The listing builds one solid part. Answer for the finished solid, in the listing's coordinates (mm). Face numbers are marked on the shaded views. A direction names the side the tool comes from. Coordinates: 2 decimals unless noted, no trailing zeros. Order: outer loops, then holes, each group sorted by start corner. A loop starts at its lowest first (then second) coordinate and runs counter-clockwise, first axis right, second up. Notation, with made-up numbers: (1, 59.25) -> (15, 59.25) arc R22 ccw to (15, 96.25) -> close; hole circle Ø9 at (21, 6.25). An arc over 180 degrees is marked (long way). Answer in a Markdown table with one row per item. Add a question column.
```python
from build123d import *

# Parameters (mm, degrees)
RESSALTO_EXTRUS_O1_DEPTH = 10
ESBO_O3_R                = 1.5
CORTE_EXTRUS_O1_DEPTH    = 10


with BuildPart() as part:
    # Esboço2 → Ressalto-extrusão1 (new body)
    with BuildSketch(Plane.XY):
        with BuildLine():
            Line((-2.16273614, 4.130820826), (4.83726386, 4.130820826))
            ThreePointArc((4.83726386, 4.130820826), (6.687556539, 1.360164653), (7.33726386, -1.907556116))
            Line((7.33726386, -1.907556116), (7.33726386, -5.469179174))
            Line((7.33726386, -5.469179174), (14.33726386, -5.469179174))
            Line((14.33726386, -5.469179174), (14.33726386, -3.493237638))
            Line((14.33726386, -3.493237638), (9.33726386, -3.493237638))
            Line((9.33726386, -3.493237638), (9.33726386, -0.739966657))
            ThreePointArc((9.33726386, -0.739966657), (8.579234613, 2.826995847), (6.436166726, 5.777434776))
            Line((6.436166726, 5.777434776), (-3.761639005, 5.777434776))
            ThreePointArc((-3.761639005, 5.777434776), (-5.904706893, 2.826995847), (-6.66273614, -0.739966657))
            Line((-6.66273614, -0.739966657), (-6.66273614, -3.493237638))
            Line((-6.66273614, -3.493237638), (-11.66273614, -3.493237638))
            Line((-11.66273614, -3.493237638), (-11.66273614, -5.469179174))
            Line((-11.66273614, -5.469179174), (-4.66273614, -5.469179174))
            Line((-4.66273614, -5.469179174), (-4.66273614, -1.907556116))
            ThreePointArc((-4.66273614, -1.907556116), (-4.013028819, 1.360164653), (-2.16273614, 4.130820826))
        make_face()
    extrude(amount=RESSALTO_EXTRUS_O1_DEPTH)

    # Esboço3 → Corte-extrusão1 (cut)
    with BuildSketch(Plane(origin=(0, -3.493237638, 0), x_dir=(1, 0, 0), z_dir=(0, 1, 0))):
        with Locations(Location((-9.16273614, -5, 0), (0, 0, 270))):
            Circle(ESBO_O3_R)
        with Locations(Location((11.83726386, -5, 0), (0, 0, 180))):
            Circle(ESBO_O3_R)
    extrude(amount=-CORTE_EXTRUS_O1_DEPTH, mode=Mode.SUBTRACT)


solid = part.part
```
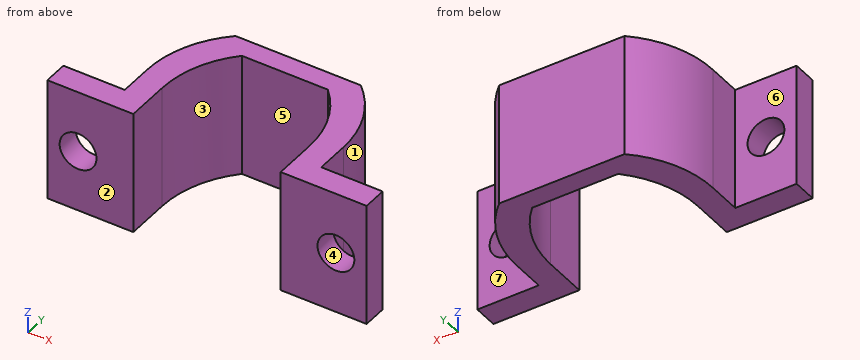
Q1. For the marked faces 4, 5, 6 and 7, determine the directions among +Z, -Z, +X, -X, +Y, -Y from which every point of the face is accessible in a straight line to the end or side of a thin tool.
Q2. A cutting plane is placed at C-C (z = 9.25). Determine the outline of the cut face in (x, y), then the cut area to 3 significant figures.
Q3. Straight lines are drawn through the part: line 1 (X direction, y = -3.25, z = 9.75); line 2 (X direction, y = -4.5, z = 8.5); line 3 (X direction, y = -4, z = 6.25). For each, find the intervals that lie inside material, in ascending order.
Q4. A cutting plane is placed at B-B (y = -3.25). Determine the outline of the cut face in (x, z).
Q5. Given pin 1 (2 mm diameter, centred on y = -1.5, z = 4, fed in from -X); pin 2 (6 mm diameter, centred on x = -1.5, y = -2.5, fed in from -Z); pin 3 (2 mm diameter, centred on y = -2, z = 6.5, fed in from +X); pin 4 (5.5 mm diameter, centred on x = -8, z = 7.5, fed in from +Y), each flat-ended and moving along its own axis, determine where each tip first touches the part or whether it passes through.
Q6. A cutting plane is placed at A-A (z = 5). Determine the outline of the cut face in (x, y), then the cut area to 3 significant figures.
Q7. A cutting plane is placed at D-D (x = -0.75). Determine the outline of the cut face in (y, z), then the cut area to 3 significant figures.
Q8. Determine the mould class of the marked faces 1, 2 and 3 for opening direction X: +X half, -X half, draft (parallel to the pull), parting line (faces both ways), or undercut.
Returned:
| question | item | result |
|---|---|---|
| 1 | face 4 | +Y, -Y |
| 1 | face 5 | +Z, -Z, -Y |
| 1 | face 6 | +Z, -Z, -X, +Y |
| 1 | face 7 | +Z, -Z, +X, +Y |
| 2 | outline | (-11.66, -5.47) -> (-4.66, -5.47) -> (-4.66, -1.91) arc R8.54 cw to (-2.16, 4.13) -> (4.84, 4.13) arc R8.54 cw to (7.34, -1.91) -> (7.34, -5.47) -> (14.34, -5.47) -> (14.34, -3.49) -> (9.34, -3.49) -> (9.34, -0.74) arc R8.77 ccw to (6.44, 5.78) -> (-3.76, 5.78) arc R8.77 ccw to (-6.66, -0.74) -> (-6.66, -3.49) -> (-11.66, -3.49) -> close |
| 2 | area | 82.3 mm² |
| 3 | line 1 | x = -6.66 to -4.66, 7.34 to 9.34 |
| 3 | line 2 | x = -11.66 to -4.66, 7.34 to 14.34 |
| 3 | line 3 | x = -11.66 to -9.99, -8.33 to -4.66, 7.34 to 11.01, 12.67 to 14.34 |
| 4 | outline | (-6.66, 0) -> (-4.66, 0) -> (-4.66, 10) -> (-6.66, 10) -> close; (7.34, 0) -> (9.34, 0) -> (9.34, 10) -> (7.34, 10) -> close |
| 5 | pin 1 | stops at x = -6.66 |
| 5 | pin 2 | passes through |
| 5 | pin 3 | stops at x = 9.34 |
| 5 | pin 4 | stops at y = 4.03 |
| 6 | outline | (-11.66, -5.47) -> (-10.66, -5.47) -> (-10.66, -3.49) -> (-11.66, -3.49) -> close; (-7.66, -5.47) -> (-4.66, -5.47) -> (-4.66, -1.91) arc R8.54 cw to (-2.16, 4.13) -> (4.84, 4.13) arc R8.54 cw to (7.34, -1.91) -> (7.34, -5.47) -> (10.34, -5.47) -> (10.34, -3.49) -> (9.34, -3.49) -> (9.34, -0.74) arc R8.77 ccw to (6.44, 5.78) -> (-3.76, 5.78) arc R8.77 ccw to (-6.66, -0.74) -> (-6.66, -3.49) -> (-7.66, -3.49) -> close; (13.34, -5.47) -> (14.34, -5.47) -> (14.34, -3.49) -> (13.34, -3.49) -> close |
| 6 | area | 70.4 mm² |
| 7 | outline | (4.13, 0) -> (5.78, 0) -> (5.78, 10) -> (4.13, 10) -> close |
| 7 | area | 16.5 mm² |
| 8 | face 1 | +X half |
| 8 | face 2 | draft |
| 8 | face 3 | undercut |
